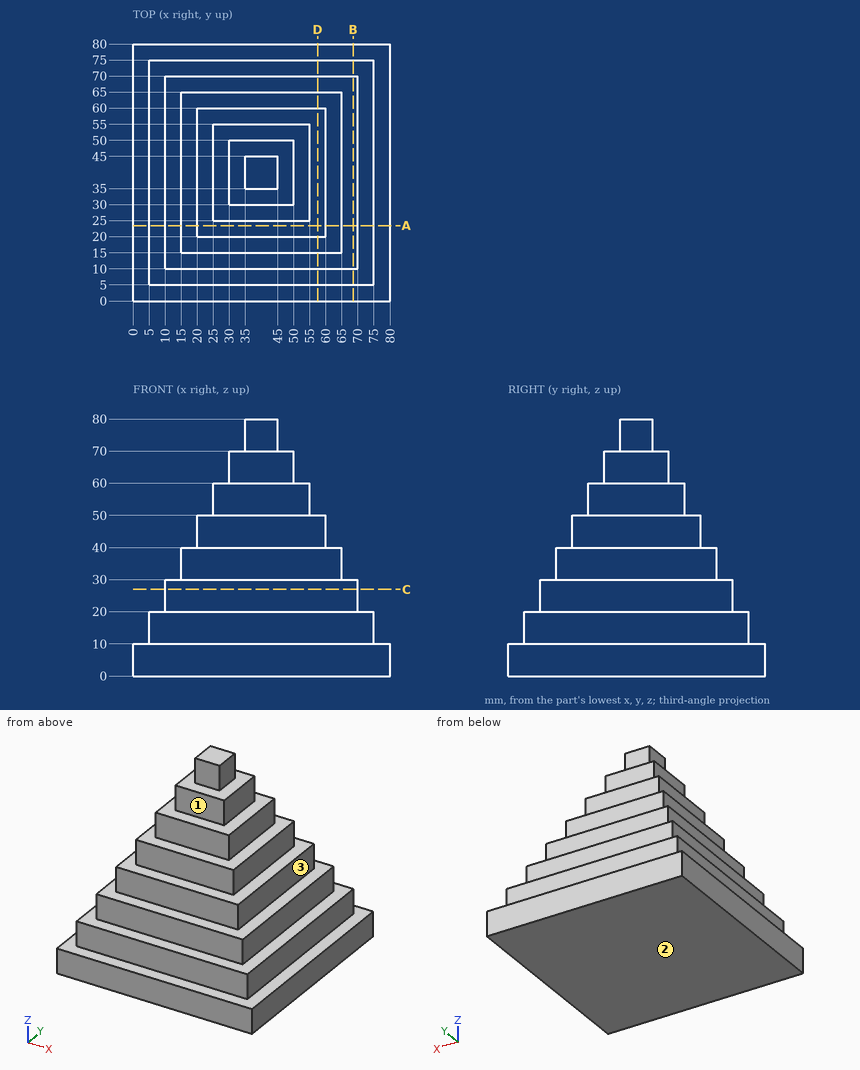
The figure shows three views and two pictorial views of one solid part (mm, origin at its lowest corner). Answer the questions. A direction names the side the tool comes from. Coordinates: 2 decimals unless noted, no trailing zeros. Write each loop counter-clockwise with the first axis right and the second up, starting at its lowest first coordinate (ties: lowest second). Pieces come first, ordered by that corner, then holes. Notation, with made-up numbers: (-12.5, 7) -> (19.5, 7) arc R19 cw to (19.5, 20) -> close; hole circle Ø9 at (33.25, -28.5). An arc over 180 degrees is marked (long way). Return JSON: item names as keys, results as strings.
(1) Each of these flat-tipped pins is pushed along its axis until it touches: P1, Ø5, axis at x = 45, z = 31, coming from the +Y side; P2, Ø3, axis at x = 44, z = 67, coming from the -Y side; P3, Ø10, axis at y = 13.5, z = 25.5, coming from the +X side; P4, Ø12, axis at x = 45.5, y = 32.5, coming from the +Z side. Where does it stop, or does it pass through?
Answers below:
{"P1": "y = 70", "P2": "y = 30", "P3": "x = 70", "P4": "z = 80"}
(2) The part is cut by section B-B on x = 68.5. Give the vertices of the cut face in (y, z).
Answers below:
{"outline": "(0, 0) -> (80, 0) -> (80, 10) -> (75, 10) -> (75, 20) -> (70, 20) -> (70, 30) -> (10, 30) -> (10, 20) -> (5, 20) -> (5, 10) -> (0, 10) -> close"}
(3) Consider line 1 along Z through (x, y) = (7.5, 16); line 2 along X through (y, z) = (28, 32); line 3 along Z through (x, y) = (10.5, 48.5). Determine where each line is inside the solid, lowest interval first. Write a range as from..to.
Answers below:
{"line 1": "0..20", "line 2": "15..65", "line 3": "0..30"}
(4) Which of the six approach directions +Z, -Z, +X, -X, +Y, -Y give full straight-line access (tool end or side, diameter ignored) to the marked faces 1, 2 and 3?
Answers below:
{"face 1": "+Z, +X, -X, -Y", "face 2": "-Z, +X, -X, +Y, -Y", "face 3": "+Z, +X, +Y, -Y"}
(5) The part is cut by section C-C on z = 27. Give the vertices of the cut face in (x, y).
Answers below:
{"outline": "(10, 10) -> (70, 10) -> (70, 70) -> (10, 70) -> close"}
(6) The part is cut by section A-A on y = 23.5. Give the vertices of the cut face in (x, z).
Answers below:
{"outline": "(0, 0) -> (80, 0) -> (80, 10) -> (75, 10) -> (75, 20) -> (70, 20) -> (70, 30) -> (65, 30) -> (65, 40) -> (60, 40) -> (60, 50) -> (20, 50) -> (20, 40) -> (15, 40) -> (15, 30) -> (10, 30) -> (10, 20) -> (5, 20) -> (5, 10) -> (0, 10) -> close"}
